CAD build for the part. Positions are in the model's coordinates, mm. A direction names the side the tool comes from. Round coordinates to 2 decimals unless told otherwise and drop trailing zeros. Loops run counter-clockwise (first coordinate to the right, second up) from the corner with the lowest first, then second, coordinate; pieces in that order, holes last. Notation, with made-up numbers: M -10.75,28.25 L 37.25,28.25 A16 cw 37.25,55.25 Z; hole C 14.5,54 d7. An arc over 180 degrees is marked long. Use one line per item in the form item = value.
from build123d import *

# Parameters (mm, degrees)
BOSS_EXTRUDE2_DEPTH                = 1.5
F_3_0_3_DIAMETER_HOLE2_D           = 3
F_3_0_3_DIAMETER_HOLE2_DEPTH       = 4
F_3_0_3_DIAMETER_HOLE2_CSINK_D     = 3.05
F_3_0_3_DIAMETER_HOLE2_CSINK_ANGLE = 90
F_3_0_3_DIAMETER_HOLE2_TIP         = 0.901290929
F_3_0_3_DIAMETER_HOLE3_D           = 3
F_3_0_3_DIAMETER_HOLE3_DEPTH       = 4
F_3_0_3_DIAMETER_HOLE3_CSINK_D     = 3.05
F_3_0_3_DIAMETER_HOLE3_CSINK_ANGLE = 90
F_3_0_3_DIAMETER_HOLE3_TIP         = 0.901290929
F_3_0_3_DIAMETER_HOLE4_D           = 3
F_3_0_3_DIAMETER_HOLE4_DEPTH       = 4
F_3_0_3_DIAMETER_HOLE4_CSINK_D     = 3.05
F_3_0_3_DIAMETER_HOLE4_CSINK_ANGLE = 90
F_3_0_3_DIAMETER_HOLE4_TIP         = 0.901290929


with BuildPart() as part:
    # Sketch1 → Boss-Extrude2 (new body)
    with BuildSketch(Plane.XY):
        with BuildLine():
            Line((0, 0), (-124, 0))
            Line((-124, 0), (-124, -38))
            ThreePointArc((-124, -38), (-123.414213562, -39.414213562), (-122, -40))
            Line((-122, -40), (-78.713430221, -40))
            ThreePointArc((-78.713430221, -40), (-76.328551688, -40.60541761), (-74.521212139, -42.275058247))
            Line((-74.521212139, -42.275058247), (-67.192218082, -53.550433721))
            ThreePointArc((-67.192218082, -53.550433721), (-63, -55.825491968), (-58.807781918, -53.550433721))
            Line((-58.807781918, -53.550433721), (-51.478787861, -42.275058247))
            ThreePointArc((-51.478787861, -42.275058247), (-49.671448312, -40.60541761), (-47.286569779, -40))
            Line((-47.286569779, -40), (-31.073173444, -40))
            ThreePointArc((-31.073173444, -40), (-30.023896938, -40.111337727), (-29.021350058, -40.440392474))
            Line((-29.021350058, -40.440392474), (-10.978649942, -48.559607526))
            ThreePointArc((-10.978649942, -48.559607526), (-9.976103062, -48.888662273), (-8.926826556, -49))
            Line((-8.926826556, -49), (58, -49))
            ThreePointArc((58, -49), (59.414213562, -49.585786438), (60, -51))
            Line((60, -51), (60, -53))
            ThreePointArc((60, -53), (60.585786438, -54.414213562), (62, -55))
            Line((62, -55), (122, -55))
            ThreePointArc((122, -55), (123.414213562, -54.414213562), (124, -53))
            Line((124, -53), (124, 0))
            Line((124, 0), (0, 0))
        make_face()
    boss_extrude2 = extrude(amount=-BOSS_EXTRUDE2_DEPTH)

    # Mirror1: Boss-Extrude2 across plane
    add(boss_extrude2.mirror(Plane(origin=(0, 0, -1.5), x_dir=(0, 0, 1), z_dir=(0, 1, 0))))

    # Ø3.0 (3) Diameter Hole2
    with Locations(Plane.XY):
        with Locations((115.95, 46), (-117, 16), (115.95, -46), (-117, -16)):
            CounterSinkHole(F_3_0_3_DIAMETER_HOLE2_D / 2, F_3_0_3_DIAMETER_HOLE2_CSINK_D / 2, depth=F_3_0_3_DIAMETER_HOLE2_DEPTH, counter_sink_angle=F_3_0_3_DIAMETER_HOLE2_CSINK_ANGLE)
            with Locations((0, 0, -(F_3_0_3_DIAMETER_HOLE2_DEPTH + F_3_0_3_DIAMETER_HOLE2_TIP / 2))):  # 118° drill point
                Cone(0, F_3_0_3_DIAMETER_HOLE2_D / 2, F_3_0_3_DIAMETER_HOLE2_TIP, mode=Mode.SUBTRACT)

    # Ø3.0 (3) Diameter Hole3
    with Locations(Plane.XY):
        with Locations((-63, 50.825491968), (-68, 40), (-58, 40), (-58, -40), (-68, -40), (-63, -50.825491968)):
            CounterSinkHole(F_3_0_3_DIAMETER_HOLE3_D / 2, F_3_0_3_DIAMETER_HOLE3_CSINK_D / 2, depth=F_3_0_3_DIAMETER_HOLE3_DEPTH, counter_sink_angle=F_3_0_3_DIAMETER_HOLE3_CSINK_ANGLE)
            with Locations((0, 0, -(F_3_0_3_DIAMETER_HOLE3_DEPTH + F_3_0_3_DIAMETER_HOLE3_TIP / 2))):  # 118° drill point
                Cone(0, F_3_0_3_DIAMETER_HOLE3_D / 2, F_3_0_3_DIAMETER_HOLE3_TIP, mode=Mode.SUBTRACT)

    # Ø3.0 (3) Diameter Hole4
    with Locations(Plane.XY):
        with Locations((100, 47.5), (70, 47.5), (70, 23.5), (100, 23.5), (100, -47.5), (100, -23.5), (70, -23.5), (70, -47.5)):
            CounterSinkHole(F_3_0_3_DIAMETER_HOLE4_D / 2, F_3_0_3_DIAMETER_HOLE4_CSINK_D / 2, depth=F_3_0_3_DIAMETER_HOLE4_DEPTH, counter_sink_angle=F_3_0_3_DIAMETER_HOLE4_CSINK_ANGLE)
            with Locations((0, 0, -(F_3_0_3_DIAMETER_HOLE4_DEPTH + F_3_0_3_DIAMETER_HOLE4_TIP / 2))):  # 118° drill point
                Cone(0, F_3_0_3_DIAMETER_HOLE4_D / 2, F_3_0_3_DIAMETER_HOLE4_TIP, mode=Mode.SUBTRACT)


solid = part.part
1. Tool access for faces 1 (the face through (-20.13, 44.44, -0.74)), 2 (the face through (-70.91, 47.83, -0.74)), 3 (the face through (-55.2, -48, -0.7)): list every direction of +Z, -Z, +X, -X, +Y, -Y with a clear straight run to the whole face (end or side of a thin tool).
Completed:
face_1 = +Z, -Z, +Y
face_2 = +Z, -Z, -X, +Y
face_3 = +Z, -Z, -Y
2. Pull direction X, two halves, no side cores. Call faces 4 (the face through (-2, -1, 0)), 5 (the face through (-55.2, 48, -0.7)), 6 (the face through (-70.91, -47.83, -0.74)): +X half, -X half, draft (parallel to the pull), parting line (faces both ways), or undercut.
Completed:
face_4 = draft
face_5 = undercut
face_6 = -X half
3. Cut at C-C on x = -90. Write the cut outline in (y, z), and give its area (3 significant figures).
Completed:
outline = M -40,-1.5 L 40,-1.5 L 40,0 L -40,0 Z
area = 120 mm2
4. Cut at A-A on x = 41. Write the cut outline in (y, z), and give its area (3 significant figures).
Completed:
outline = M -49,-1.5 L 49,-1.5 L 49,0 L -49,0 Z
area = 147 mm2
5. Drop flat-ended pins along their axis: P1, Ø2.5, axis at x = 70, y = 47.5, coming from the +Z side; P2, Ø4, axis at x = 100, y = -23.5, coming from the +Z side; P3, Ø0.8, axis at x = -40.5, z = -1, coming from the +Y side. Give the stop position or say it passes through.
Completed:
P1 = through
P2 = 0
P3 = 40
6. Probe line 1 along Y through (x, z) = (-58, -0.65); line 2 along Y through (x, z) = (100, -0.6); line 3 along Y through (x, z) = (-117, -1). List the from-to ranges inside material, lowest first. Write a range as from..to.
Completed:
line_1 = -52.31..-41.5, -38.5..38.5, 41.5..52.31
line_2 = -55..-49, -46..-25, -22..22, 25..46, 49..55
line_3 = -40..-17.5, -14.5..14.5, 17.5..40
7. Cut at B-B on z = -0.6. State how many separate pieces and enclosed holes the cut face has, and give its area (3 significant figures).
Completed:
separate_pieces = 1
enclosed_holes = 18
area = 23,600 mm2
